Design review of the part built by this model. Coordinates are the model's own, in mm. Face numbers are marked on the shaded views. A direction names the side the tool comes from. Coordinates: 2 decimals unless noted, no trailing zeros. Loops run counter-clockwise (first coordinate to the right, second up) from the corner with the lowest first, then second, coordinate; pieces in that order, holes last. Notation, with made-up numbers: (43.25, 73.5) -> (51.25, 73.5) arc R25 ccw to (51.25, 104.5) -> close; hole circle Ø3 at (56, 41.25). An arc over 180 degrees is marked (long way). Answer in a Markdown table with one row per item.
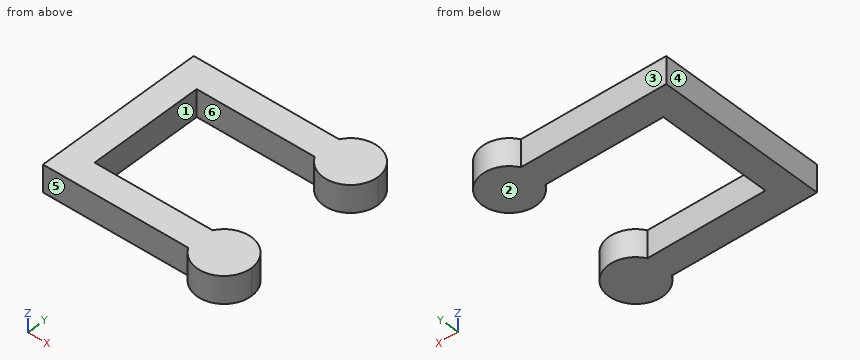
```python
from build123d import *

# Parameters (mm, degrees)
F2_DEPTH = 5


with BuildPart() as f2:
    # F1 (on Top) → F2 (new body)
    with BuildSketch(Plane.XY):
        Polygon((-10.5, -10.5), (-10.5, 10.5), (-15.5, 10.5), (-15.5, -15.5), (-10.5, -15.5), align=None)
        with BuildLine():
            Line((-10.5, 10.5), (10.5, 10.5))
            Line((10.5, 10.5), (11.1698729811, 10.5))
            ThreePointArc((11.1698729811, 10.5), (10.5, 13), (11.1698729811, 15.5))
            Line((11.1698729811, 15.5), (-15.5, 15.5))
            Line((-15.5, 15.5), (-15.5, 10.5))
            Line((-15.5, 10.5), (-10.5, 10.5))
        make_face()
        with BuildLine():
            ThreePointArc((11.1698729811, 15.5), (10.5, 13), (11.1698729811, 10.5))
            Line((11.1698729811, 10.5), (15.5, 10.5))
            Line((15.5, 10.5), (15.5, 15.5))
            Line((15.5, 15.5), (11.1698729811, 15.5))
        make_face()
        with BuildLine():
            Line((15.5, 10.5), (11.1698729811, 10.5))
            ThreePointArc((11.1698729811, 10.5), (16.7940952255, 8.1703708686), (20.5, 13))
            ThreePointArc((20.5, 13), (16.7940952255, 17.8296291314), (11.1698729811, 15.5))
            Line((11.1698729811, 15.5), (15.5, 15.5))
            Line((15.5, 15.5), (15.5, 10.5))
        make_face()
        with BuildLine():
            Line((11.1698729811, -10.5), (10.5, -10.5))
            Line((10.5, -10.5), (-10.5, -10.5))
            Line((-10.5, -10.5), (-10.5, -15.5))
            Line((-10.5, -15.5), (11.1698729811, -15.5))
            ThreePointArc((11.1698729811, -15.5), (10.5, -13), (11.1698729811, -10.5))
        make_face()
        with BuildLine():
            Line((15.5, -10.5), (11.1698729811, -10.5))
            ThreePointArc((11.1698729811, -10.5), (10.5, -13), (11.1698729811, -15.5))
            Line((11.1698729811, -15.5), (15.5, -15.5))
            Line((15.5, -15.5), (15.5, -10.5))
        make_face()
        with BuildLine():
            ThreePointArc((20.5, -13), (16.7940952255, -8.1703708686), (11.1698729811, -10.5))
            Line((11.1698729811, -10.5), (15.5, -10.5))
            Line((15.5, -10.5), (15.5, -15.5))
            Line((15.5, -15.5), (11.1698729811, -15.5))
            ThreePointArc((11.1698729811, -15.5), (16.7940952255, -17.8296291314), (20.5, -13))
        make_face()
    extrude(amount=F2_DEPTH)


solid = f2.part
```
(1) To check wall thickness, follow probe 1 along Y at (x, z) = (9, 3.5); probe 2 along X at (y, z) = (-6.5, 0.45); probe 3 along Y at (x, z) = (-14, 2.25). State the ranges of each line that lie inside material, in increasing order.
Evaluation:
| item | result |
|---|---|
| probe 1 | y = -15.5 to -10.5, 10.5 to 15.5 |
| probe 2 | x = -15.5 to -10.5 |
| probe 3 | y = -15.5 to 15.5 |
(2) For pin 1 (1.5 mm diameter, centred on x = -4, z = 1.5, fed in from +Y); pin 2 (2.5 mm diameter, centred on x = 0, z = 3.5, fed in from -Y); pin 3 (1.5 mm diameter, centred on y = -5, z = 1.5, fed in from +X), all flat-tipped, find the tip position at first contact; note any pin that passes through.
Evaluation:
| item | result |
|---|---|
| pin 1 | stops at y = 15.5 |
| pin 2 | stops at y = -15.5 |
| pin 3 | stops at x = -10.5 |
(3) Tool access review of the marked faces 1, 2 and 3: name each direction out of +Z, -Z, +X, -X, +Y, -Y from which nothing blocks a thin tool from reaching the whole face with its end or side.
Evaluation:
| item | result |
|---|---|
| face 1 | +Z, -Z |
| face 2 | -Z, +X, -X, +Y, -Y |
| face 3 | +Z, -Z, -X, +Y |
(4) Draft analysis for pull direction Y (two halves, no side actions). For the marked faces 4, 5 and 6, state which applies: pulls with the +Y half, pulls with the -Y half, needs draft (parallel to the pull), parting line crosses it, or undercut.
Evaluation:
| item | result |
|---|---|
| face 4 | needs draft |
| face 5 | pulls with the -Y half |
| face 6 | undercut |
(5) Take a section at A-A on x = -2. Give the boundary of the cut face in (y, z).
Evaluation:
| item | result |
|---|---|
| outline | (-15.5, 0) -> (-10.5, 0) -> (-10.5, 5) -> (-15.5, 5) -> close; (10.5, 0) -> (15.5, 0) -> (15.5, 5) -> (10.5, 5) -> close |
(6) Take a section at B-B on z = 1.1. Give the boundary of the cut face in (x, y), and give its area (3 significant figures).
Evaluation:
| item | result |
|---|---|
| outline | (-15.5, -15.5) -> (11.17, -15.5) arc R5 ccw (long way) to (11.17, -10.5) -> (-10.5, -10.5) -> (-10.5, 10.5) -> (11.17, 10.5) arc R5 ccw (long way) to (11.17, 15.5) -> (-15.5, 15.5) -> close |
| area | 524 mm² |
(7) Take a section at C-C on y = -9.5. Give the boundary of the cut face in (x, z), and give its area (3 significant figures).
Evaluation:
| item | result |
|---|---|
| outline | (-15.5, 0) -> (-10.5, 0) -> (-10.5, 5) -> (-15.5, 5) -> close; (11.93, 0) -> (19.07, 0) -> (19.07, 5) -> (11.93, 5) -> close |
| area | 60.7 mm² |
